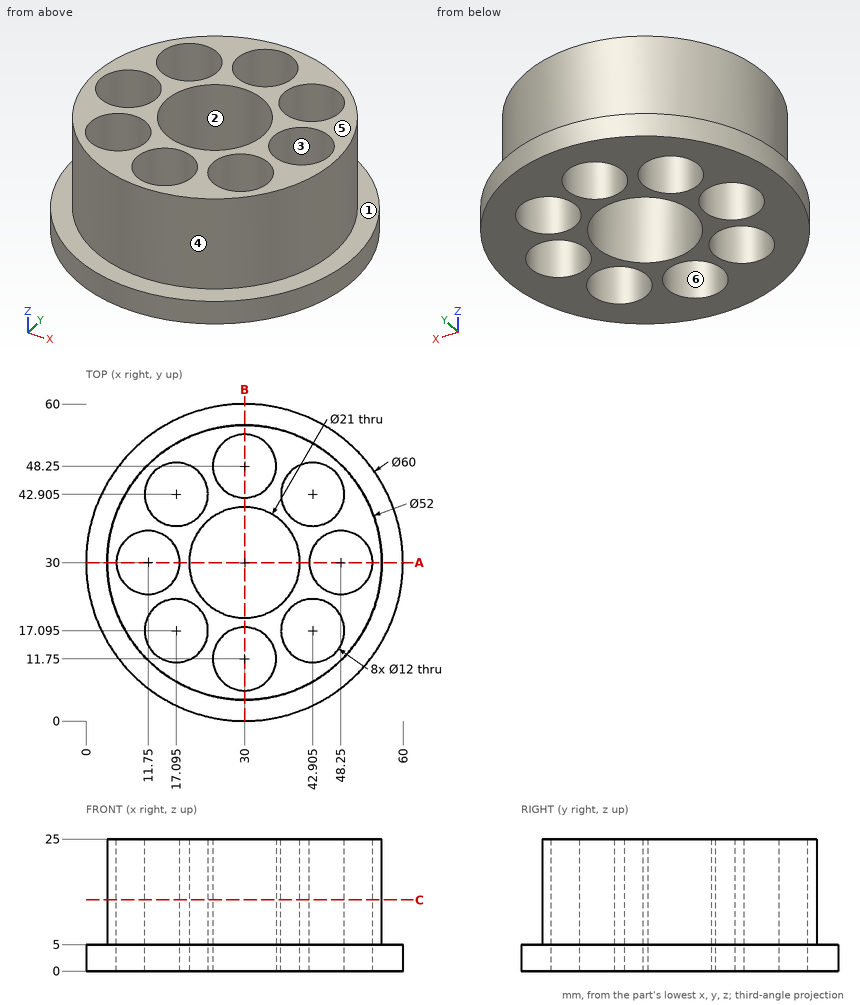
Check sheet for the drawn part. Datum: minimum x, y, z corner. Units: mm. A direction names the side the tool comes from. Round coordinates to 2 decimals unless told otherwise and drop trailing zeros. Loops run counter-clockwise (first coordinate to the right, second up) from the corner with the lowest first, then second, coordinate; pieces in that order, holes last.
Item 1: Cross-section at C-C on z = 13.5. Count the separate pieces of the cut face and the enclosed holes in it.
Item 2: Mould release check, pull along Y, two halves, no side actions. Record for the marked faces 3, 4, 5 and 6: pulls with the +Y half, pulls with the -Y half, needs draft (parallel to the pull), parting line crosses it, or undercut.
Item 3: Thickness scan on line 1 (X direction, y = 41, z = 3) (1 decimal); line 2 (Y direction, x = 15, z = 14) (1 decimal). Record the ranges inside material, lowest first.
Item 4: Access from +Z, -Z, +X, -X, +Y, -Y to the whole of each face (thin tool, end or side, straight path). Record for the marked faces 1 and 2.
Item 5: Gauge pin test, flat ends, axial feed: pin 1 (19 mm diameter, centred on x = 30, y = 11.75, fed in from +Z); pin 2 (10 mm diameter, centred on y = 39, z = 15, fed in from -X); pin 3 (3 mm diameter, centred on x = 45, z = 20, fed in from +Y); pin 4 (5 mm diameter, centred on y = 16, z = 12.5, fed in from +X). Record the tip position at first contact, or that the pin passes through.
Item 6: Cross-section at A-A on y = 30. Record the boundary of the cut face in (x, z), then the cut area to 3 significant figures.
Answer sheet:
1. separate pieces: 1
1. enclosed holes: 9
2. face 3: undercut
2. face 4: parting line crosses it
2. face 5: needs draft
2. face 6: undercut
3. line 1: x = 2.1 to 11.4, 22.8 to 37.2, 48.6 to 57.9
3. line 2: y = 8.8 to 11.5, 22.7 to 25, 35 to 37.3, 48.5 to 51.2
4. face 1: +Z
4. face 2: +Z, -Z
5. pin 1: stops at z = 25
5. pin 2: stops at x = 4.31
5. pin 3: stops at y = 52.22
5. pin 4: stops at x = 53.32
6. outline: (0, 0) - (5.75, 0) - (5.75, 25) - (4, 25) - (4, 5) - (0, 5) - close; (17.75, 0) - (19.5, 0) - (19.5, 25) - (17.75, 25) - close; (40.5, 0) - (42.25, 0) - (42.25, 25) - (40.5, 25) - close; (54.25, 0) - (60, 0) - (60, 5) - (56, 5) - (56, 25) - (54.25, 25) - close
6. area: 215 mm2
